Could you check a few things on this model? Use its own coordinates, in mm. Coordinates: 2 decimals unless noted, no trailing zeros. Loops run counter-clockwise (first coordinate to the right, second up) from the corner with the lowest first, then second, coordinate; pieces in that order, holes last. Notation, with made-up numbers: (-24, 21) - (12, 21) arc R28 cw to (12, 44) - close; hole circle Ø11 at (-2, -5). An arc over 180 degrees is marked (long way). Use CSV: the item, a comma, the result in double quotes.
from build123d import *

# Parameters (mm, degrees)
F1_DEPTH = 3
F2_D     = 2.5
F3_D     = 2.5


with BuildPart() as f1:
    # F0 (on Top) → F1 (new body)
    with BuildSketch(Plane.XY):
        with BuildLine():
            Line((-3.613195, 4.974902), (-4.113541, 0))
            Line((-4.113541, 0), (-3.613195, -4.974902))
            ThreePointArc((-3.613195, -4.974902), (0, -8.242932), (3.613195, -4.974902))
            Line((3.613195, -4.974902), (4.113541, 0))
            Line((4.113541, 0), (3.613195, 4.974902))
            ThreePointArc((3.613195, 4.974902), (0, 8.242932), (-3.613195, 4.974902))
        make_face()
    extrude(amount=F1_DEPTH)

    # F2 (through all)
    with Locations(Plane(origin=(0, 0, 0), x_dir=(1, 0, 0), z_dir=(0, 0, -1))):
        with Locations((0, 4.611509)):
            Hole(F2_D / 2)

    # F3 (through all)
    with Locations(Plane(origin=(0, 0, 0), x_dir=(1, 0, 0), z_dir=(0, 0, -1))):
        with Locations((0, -4.611509)):
            Hole(F3_D / 2)


solid = f1.part
(1) Suppose I cut it at D-D (x = 2.5). Write out the boundary of the cut face in (y, z).
Computed:
outline,"(-7.25, 0) - (7.25, 0) - (7.25, 3) - (-7.25, 3) - close"
(2) Suppose I cut it at B-B (y = 5.25). Write out the boundary of the cut face in (x, z).
Computed:
outline,"(-3.57, 0) - (-1.07, 0) - (-1.07, 3) - (-3.57, 3) - close; (1.07, 0) - (3.57, 0) - (3.57, 3) - (1.07, 3) - close"
(3) Thinking about a two-plate mould opening in X: for faces 1 (the face through (0, 0, 3)), 2 (the face through (0.99, -3.85, 1.52)), 3 (the face through (3.867, 2.453, 1.479)), which applies, +X half, -X half, draft (parallel to the pull), parting line (faces both ways), or undercut?
Computed:
face 1,"draft"
face 2,"undercut"
face 3,"+X half"
(4) Please list where these lines run through material, in increasing order: line 1 (Y direction, x = 0, z = 1.7); line 2 (Y direction, x = -0.25, z = 1.2); line 3 (X direction, y = -3.75, z = 2.4).
Computed:
line 1,"y = -8.24 to -5.86, -3.36 to 3.36, 5.86 to 8.24"
line 2,"y = -8.23 to -5.84, -3.39 to 3.39, 5.84 to 8.23"
line 3,"x = -3.74 to -0.91, 0.91 to 3.74"
(5) Suppose I cut it at A-A (x = 0). Write out the boundary of the cut face in (y, z), plus the area to 3 significant figures.
Computed:
outline,"(-8.24, 0) - (-5.86, 0) - (-5.86, 3) - (-8.24, 3) - close; (-3.36, 0) - (3.36, 0) - (3.36, 3) - (-3.36, 3) - close; (5.86, 0) - (8.24, 0) - (8.24, 3) - (5.86, 3) - close"
area,"34.5 mm²"
(6) Suppose I cut it at C-C (z = 2.4). Write out the boundary of the cut face in (x, y), plus the area to 3 significant figures.
Computed:
outline,"(-4.11, 0) - (-3.61, -4.97) arc R3.63 ccw to (3.61, -4.97) - (4.11, 0) - (3.61, 4.97) arc R3.63 ccw to (-3.61, 4.97) - close; hole circle Ø2.5 at (0, -4.61); hole circle Ø2.5 at (0, 4.61)"
area,"103 mm²"
(7) Will these pins go through, and if not, where does the flat tip stop? pin 1 (1.5 mm diameter, centred on x = 1, z = 1.5, fed in from +Y); pin 2 (3 mm diameter, centred on x = 0, y = 4.61, fed in from -Z); pin 3 (1.5 mm diameter, centred on x = 3, z = 1, fed in from +Y).
Computed:
pin 1,"stops at y = 8.23"
pin 2,"stops at z = 0"
pin 3,"stops at y = 7.46"
